```python
from build123d import *

# Parameters (mm, degrees)
PAD044_DEPTH    = 42
SKETCH127_R     = 1.75
SKETCH127_R_2   = 11.1
POCKET039_DEPTH = 36.001
SKETCH128_R     = 2.75
HOLE027_DEPTH   = 25
SKETCH130_W     = 25
SKETCH130_H     = 10
POCKET040_DEPTH = 13


with BuildPart() as part:
    # Sketch124 → Pad044 (new body)
    with BuildSketch(Plane.YZ):
        Polygon((-32, 10), (-32, 43), (10, 43), (10, 10), (33, 10), (33, 13), (13, 13), (13, 46), (-35, 46), (-35, 13), (-65, 13), (-65, 10), align=None)
    extrude(amount=PAD044_DEPTH)

    # Sketch127 (on Face8 of Pad044) → Pocket039 (cut, through all)
    with BuildSketch(Plane(origin=(0, 0, 46), x_dir=(0, -1, 0), z_dir=(0, 0, 1))):
        with Locations((-4.5, 36.5)):
            Circle(SKETCH127_R)
        with Locations((-4.5, 5.5)):
            Circle(SKETCH127_R)
        with Locations((26.5, 36.5)):
            Circle(SKETCH127_R)
        with Locations((26.5, 5.5)):
            Circle(SKETCH127_R)
        with Locations((11, 21)):
            Circle(SKETCH127_R_2)
    extrude(amount=-POCKET039_DEPTH, mode=Mode.SUBTRACT)

    # Sketch128 (on Face19 of Pocket039) → Hole027 (cut)
    with BuildSketch(Plane(origin=(0, 0, 13), x_dir=(0, -1, 0), z_dir=(0, 0, 1))):
        with Locations((55, 31)):
            Circle(SKETCH128_R)
        with Locations((55, 11)):
            Circle(SKETCH128_R)
    extrude(amount=-HOLE027_DEPTH, mode=Mode.SUBTRACT)

    # Sketch130 → Pocket040 (cut)
    with BuildSketch(Plane.XZ.offset(40)):
        with Locations((21, 15)):
            Rectangle(SKETCH130_W, SKETCH130_H)
    extrude(amount=-POCKET040_DEPTH, mode=Mode.SUBTRACT)


with BuildPart() as part_1:
    # Body019 placement: moved
    add(part.part.moved(Location((-21, 0, 0))))


solid = part_1.part
```
The model under review builds one solid part; all positions refer to its coordinate system, in mm. A direction names the side the tool comes from. Round coordinates to 2 decimals unless told otherwise and drop trailing zeros. Order: outer loops, then holes, each group sorted by start corner. A loop starts at its lowest first (then second) coordinate and runs counter-clockwise, first axis right, second up. Notation, with made-up numbers: (59.5, 36.25) -> (115.5, 36.25) arc R24 ccw to (115.5, 57.25) -> close; hole circle Ø10 at (87.5, 80). An arc over 180 degrees is marked (long way). Use a Markdown table: item, result.
Q1. We need section B-B on x = -15.5. Write out the cut boundary in (y, z).
Values:
| item | result |
|---|---|
| outline | (-65, 10) -> (-32, 10) -> (-32, 43) -> (-28.25, 43) -> (-28.25, 46) -> (-35, 46) -> (-35, 13) -> (-65, 13) -> close; (-24.75, 43) -> (2.75, 43) -> (2.75, 46) -> (-24.75, 46) -> close; (6.25, 43) -> (10, 43) -> (10, 10) -> (33, 10) -> (33, 13) -> (13, 13) -> (13, 46) -> (6.25, 46) -> close |
Q2. We need section A-A on y = -55. Write out the cut boundary in (x, z).
Values:
| item | result |
|---|---|
| outline | (-21, 10) -> (-12.75, 10) -> (-12.75, 13) -> (-21, 13) -> close; (-7.25, 10) -> (7.25, 10) -> (7.25, 13) -> (-7.25, 13) -> close; (12.75, 10) -> (21, 10) -> (21, 13) -> (12.75, 13) -> close |
Q3. Mouldability with a two-part tool opening along X and no side actions: class faces 1 (the flat face through (0, -40, 12)), 2 (the flat face through (0, -32, 30)), 3 (the flat face through (21, -13, 44)) as +X half, -X half, draft (parallel to the pull), parting line (faces both ways), or undercut.
Values:
| item | result |
|---|---|
| face 1 | undercut |
| face 2 | draft |
| face 3 | +X half |
Q4. Tool access review of faces 4 (the flat face through (0, 13, 29)), 5 (the flat face through (-12.5, -34, 14)), 6 (the flat face through (0, -34, 20)), 7 (the flat face through (0, -35, 30)): name each direction out of +Z, -Z, +X, -X, +Y, -Y from which nothing blocks a thin tool from reaching the whole face with its end or side.
Values:
| item | result |
|---|---|
| face 4 | +Z, +X, -X, +Y |
| face 5 | -Z |
| face 6 | -Z, -Y |
| face 7 | +Z, +X, -X, -Y |
Q5. For line 1 (X direction, y = -26.5, z = 45.4); line 2 (Y direction, x = -10, z = 26.5); line 3 (X direction, y = -11, z = 45), list the stretches that pass through material, from the lowest coordinate up.
Values:
| item | result |
|---|---|
| line 1 | x = -21 to -17.25, -13.75 to 13.75, 17.25 to 21 |
| line 2 | y = -35 to -32, 10 to 13 |
| line 3 | x = -21 to -11.1, 11.1 to 21 |
Q6. Clearance check with flat-ended pins moving along their axes: P1, Ø12.5, axis at x = -6.5, y = -14.5, coming from the -Z side; P2, Ø1.5, axis at x = -11.5, y = -34, coming from the -Z side; P3, Ø16.5, axis at x = -5.5, z = 34, coming from the -Y side. State where each tip first meets the part, or that it passes through.
Values:
| item | result |
|---|---|
| P1 | stops at z = 43 |
| P2 | stops at z = 20 |
| P3 | stops at y = -35 |
Q7. We need section C-C on z = 14. Write out the cut boundary in (x, y).
Values:
| item | result |
|---|---|
| outline | (-21, -35) -> (-12.5, -35) -> (-12.5, -32) -> (-21, -32) -> close; (-21, 10) -> (21, 10) -> (21, 13) -> (-21, 13) -> close; (12.5, -35) -> (21, -35) -> (21, -32) -> (12.5, -32) -> close |
Q8. We need section D-D on y = -11. Write out the cut boundary in (x, z), then the cut area to 3 significant figures.
Values:
| item | result |
|---|---|
| outline | (-21, 43) -> (-11.1, 43) -> (-11.1, 46) -> (-21, 46) -> close; (11.1, 43) -> (21, 43) -> (21, 46) -> (11.1, 46) -> close |
| area | 59.4 mm^2 |
